Geometry: final body of the model. Coordinates: model frame, mm. A direction names the side the tool comes from. Round coordinates to 2 decimals unless told otherwise and drop trailing zeros. Loops run counter-clockwise (first coordinate to the right, second up) from the corner with the lowest first, then second, coordinate; pieces in that order, holes last. Notation, with made-up numbers: M 58.5,35.5 L 82.5,35.5 A27 ccw 82.5,63.5 Z; hole C -19.75,63.25 d3. An arc over 180 degrees is marked long. Return JSON: item names as keys, results as strings.
Autodesk Inventor part; units mm, degrees
ref_plane "YZ Plane" through (0, 0, 0) normal (1, 0, 0) x (0, 1, 0)
ref_plane "XZ Plane" through (0, 0, 0) normal (0, 1, 0) x (-1, 0, 0)
ref_plane "XY Plane" through (0, 0, 0) normal (0, 0, 1) x (1, 0, 0)
sketch "Sketch1" plane through (0, 0, 0) normal (0, 0, 1) x (1, 0, 0)
  line L0 (-12.2, -17.05) -> (12.2, -17.05)
  line L1 (12.2, -17.05) -> (12.2, 17.05)
  line L2 (12.2, 17.05) -> (-12.2, 17.05)
  line L3 (-12.2, 17.05) -> (-12.2, -17.05)
  line L4 (-12.2, -17.05) -> (12.2, 17.05) construction
  line L5 (12.2, -17.05) -> (-12.2, 17.05) construction
  circle A0 centre (-10, 14.92) radius 1.5
  circle A1 centre (10, 14.92) radius 1.5
  line L6 (-10, 14.92) -> (10, 14.92) construction
  circle A2 centre (-9, 9.05) radius 0.8
  circle A3 centre (-10, 9.05) radius 0.8
  circle A4 centre (9, 9.05) radius 0.8
  circle A5 centre (10, 9.05) radius 0.8
  line L7 (-9, 9.05) -> (9, 9.05) construction
  line L8 (-10, 9.05) -> (10, 9.05) construction
  point P0 (0, 0)
  point P1 (0, 9.05)
  point P2 (0, 14.92)
  point P3 (0, 0)
  point P4 (0, 0)
  dimension "d0" = 24.4
  dimension "d1" = 34.1
  dimension "d2" = 2.13
  dimension "d3" = 3
  dimension "d4" = 10
  dimension "d13" = 20
  dimension "d14" = 18
  dimension "d15" = 1.6
  dimension "d16" = 8
extrude "Extrusion1" add sketch "Sketch1" along normal mid plane 1.6
sketch "Sketch2" plane through (0, 0, -0.8) normal (0, 0, -1) x (-1, 0, 0)
  circle A0 centre (-10, 14.92) radius 1.5
  circle A1 centre (10, 14.92) radius 1.5
  line L0 (-12.2, -17.05) -> (12.2, -17.05)
  line L1 (12.2, -17.05) -> (12.2, 17.05)
  line L2 (12.2, 17.05) -> (-12.2, 17.05)
  line L3 (-12.2, 17.05) -> (-12.2, -17.05)
  line L4 (-10.16, -12.99) -> (10.16, -12.99)
  line L5 (10.16, -12.99) -> (10.16, -15.53)
  line L6 (10.16, -15.53) -> (-10.16, -15.53)
  line L7 (-10.16, -15.53) -> (-10.16, -12.99)
  point P0 (0, 0)
  point P1 (0, -12.99)
  point P2 (-10.16, -14.26)
  dimension "d8" = 2.54
  dimension "d9" = 20.32
  dimension "d10" = 2.79
extrude "Extrusion2" add sketch "Sketch2" against normal blind 4.1 contours L4 L5 L6 L7
sketch "Sketch3" plane through (0, 0, 0.8) normal (0, 0, 1) x (1, 0, 0)
  circle A0 centre (10, 14.92) radius 1.5
  circle A1 centre (-10, 14.92) radius 1.5
  arc A2 (-9.5, 8.4255) -> (-9.5, 9.6745) centre (-9, 9.05) ccw
  arc A3 (-9.5, 9.6745) -> (-9.5, 8.4255) centre (-10, 9.05) ccw
  line L0 (-12.2, -17.05) -> (12.2, -17.05)
  line L1 (12.2, -17.05) -> (12.2, 17.05)
  line L2 (12.2, 17.05) -> (-12.2, 17.05)
  line L3 (-12.2, 17.05) -> (-12.2, -17.05)
  arc A4 (9.5, 9.6745) -> (9.5, 8.4255) centre (9, 9.05) ccw
  arc A5 (9.5, 8.4255) -> (9.5, 9.6745) centre (10, 9.05) ccw
  line L4 (-3.4725, 12.5225) -> (3.4725, 12.5225)
  line L5 (3.4725, 12.5225) -> (3.4725, 5.5775)
  line L6 (3.4725, 5.5775) -> (-3.4725, 5.5775)
  line L7 (-3.4725, 5.5775) -> (-3.4725, 12.5225)
  point P0 (0, 0)
  point P1 (3.4725, 9.05)
  point P2 (0, 12.5225)
  dimension "d17" = 6.945
extrude "Extrusion3" add sketch "Sketch3" along normal blind 0.78 contours L4 L5 L6 L7
sketch "Sketch4" plane through (0, 0, 1.58) normal (0, 0, 1) x (1, 0, 0)
  line L0 (3.4725, 12.5225) -> (-3.4725, 12.5225)
  line L1 (-3.4725, 12.5225) -> (-3.4725, 5.5775)
  line L2 (-3.4725, 5.5775) -> (3.4725, 5.5775)
  line L3 (3.4725, 5.5775) -> (3.4725, 12.5225)
  circle A0 centre (0, 9.05) radius 3.175
  point P0 (0, 0)
  point P1 (0, 12.5225)
  point P2 (-3.4725, 9.05)
  dimension "d20" = 6.35
extrude "Extrusion4" cut sketch "Sketch4" against normal blind 0.1 contours A0
equation "\"d9\" = 8 * d8"
properties part number "Module_ArducamMini-Rev" material "Epoxy Resin"
Q1. Reachability of faces 5 (the flat face through (0, 9, 1.48)), 6 (the flat face through (-10.16, -14, 2)), 7 (the flat face through (0, 0, -0.8)), 8 (the flat face through (10.16, -14, 2)), 9 (the flat face through (0, -15.53, 2)) from +Z, -Z, +X, -X, +Y, -Y: full face, straight path, thin tool, end or side. Return the list, or none.
Determined:
{"face 5": "+Z", "face 6": "+Z, -X, +Y, -Y", "face 7": "-Z, +X, -X, +Y, -Y", "face 8": "+Z, +X, +Y, -Y", "face 9": "+Z, +X, -X, -Y"}
Q2. Section query D-D (z = -0.25). Output: boundary loops of the cut face in (x, y).
Determined:
{"outline": "M -12.2,-17.05 L 12.2,-17.05 L 12.2,17.05 L -12.2,17.05 Z; hole C -10,14.92 d3; hole M -9.5,8.43 A0.8 ccw long -9.5,9.67 A0.8 ccw long Z; hole C 10,14.92 d3; hole M 9.5,8.43 A0.8 ccw long 9.5,9.67 A0.8 ccw long Z"}
Q3. Pull-direction query (X, two-part tool) for faces 1 (the flat face through (0, -14, 3.3)), 2 (the cylindrical face through (8.2, 9, 0)), 3 (the flat face through (12.2, 0, 0)), 4 (the cylindrical face through (9.805, 13.433, -0.011)); classes: pulls with the +X half, pulls with the -X half, needs draft (parallel to the pull), parting line crosses it, or undercut.
Determined:
{"face 1": "needs draft", "face 2": "undercut", "face 3": "pulls with the +X half", "face 4": "undercut"}
Q4. Section query C-C (x = -9). Output: boundary loops of the cut face in (y, z).
Determined:
{"outline": "M -17.05,-0.8 L 8.25,-0.8 L 8.25,0.8 L -12.99,0.8 L -12.99,3.3 L -15.53,3.3 L -15.53,0.8 L -17.05,0.8 Z; M 9.85,-0.8 L 13.8,-0.8 L 13.8,0.8 L 9.85,0.8 Z; M 16.04,-0.8 L 17.05,-0.8 L 17.05,0.8 L 16.04,0.8 Z"}
Q5. Pin query (flat end, axial travel): pin 1 (1.5 mm diameter, centred on y = -12.5, z = 2.5, fed in from +X); pin 2 (2.5 mm diameter, centred on x = 10, y = 14.92, fed in from -Z); pin 3 (4 mm diameter, centred on x = -3, y = 6.5, fed in from +Z); pin 4 (1 mm diameter, centred on x = -5, z = 2.5, fed in from +Y). Return the tip coordinate at first contact, or that it passes through.
Determined:
{"pin 1": "stops at x = 10.16", "pin 2": "passes through", "pin 3": "stops at z = 1.58", "pin 4": "stops at y = -12.99"}
Q6. Material intervals for L1, parallel to Y at x = 10, z = -0.05; L2, parallel to Y at x = 9, z = 0.4; L3, parallel to Y at x = -4.5, z = 2.3, sorted ascending.
Determined:
{"L1": "y = -17.05 to 8.25, 9.85 to 13.42, 16.42 to 17.05", "L2": "y = -17.05 to 8.25, 9.85 to 13.8, 16.04 to 17.05", "L3": "y = -15.53 to -12.99"}
Q7. Section query A-A (y = 9.05). State how many separate pieces and enclosed holes the cut face has, plus the area to 3 significant figures.
Determined:
{"separate pieces": "3", "enclosed holes": "0", "area": "35.5 mm^2"}
